from build123d import *

# Parameters (mm, degrees)
SKETCH_1_R      = 3
EXTRUDE_1_DEPTH = 5


with BuildPart() as part:
    # 草图1 → 凸台-拉伸1 (new body)
    with BuildSketch(Plane(origin=(0, 0, 0), x_dir=(1, 0, 0), z_dir=(0, 1, 0))):
        with BuildLine():
            Line((-39.885379482, -89.051728746), (240.960836827, -260.037504895))
            ThreePointArc((240.960836827, -260.037504895), (227.643725358, 34.228528193), (-39.885379482, -89.051728746))
        make_face()
        with Locations(Location((20.435189142, -16.402343887, 0), (0, 0, 270))):
            Circle(SKETCH_1_R, mode=Mode.SUBTRACT)
        with Locations(Location((-9.564810858, -68.363868114, 0), (0, 0, 270))):
            Circle(SKETCH_1_R, mode=Mode.SUBTRACT)
        with Locations(Location((250.242810277, -218.363868114, 0), (0, 0, 270))):
            Circle(SKETCH_1_R, mode=Mode.SUBTRACT)
        with Locations(Location((280.242810277, -166.402343887, 0), (0, 0, 270))):
            Circle(SKETCH_1_R, mode=Mode.SUBTRACT)
    extrude(amount=EXTRUDE_1_DEPTH)


solid = part.part
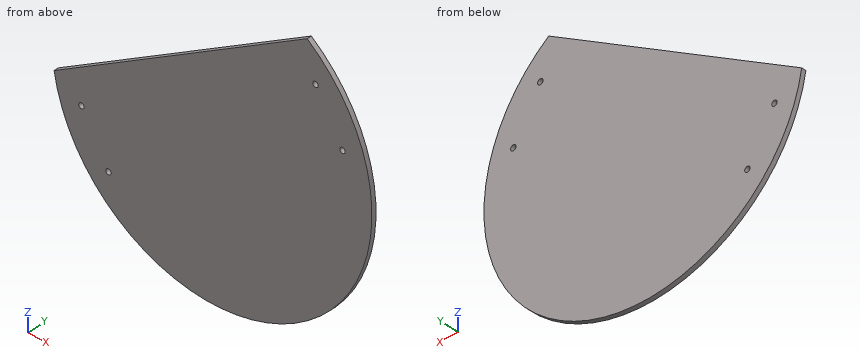
The listing builds one solid part. Answer for the finished solid, in the listing's coordinates (mm). Coordinates: 2 decimals unless noted, no trailing zeros. Loops run counter-clockwise (first coordinate to the right, second up) from the corner with the lowest first, then second, coordinate; pieces in that order, holes last.
1) Flat-ended cylindrical pins translate along their axes: pin 1 Ø2 at (x, y) = (210.5, 4) entering from +Z; pin 2 Ø3 at (x, y) = (146, 2.5) entering from -Z; pin 3 Ø2 at (x, y) = (78.5, 2.5) entering from -Z. Find the tip coordinate at first contact, or state that the pin passes through.
2) Find section A-A on y = 1.75. Write down the section's boundary in (x, z).
3) Find section C-C on z = 104.5. Write down the section's boundary in (x, y), then the cut area to 3 significant figures.
4) Find section B-B on x = 237. Write down the section's boundary in (y, z).
5) Find the intervals of material crossed by L1, parallel to Z at x = 29, y = 1.45; L2, parallel to X at y = 4.3, z = 68.5; L3, parallel to Z at x = 278, y = 1.05, in increasing order.
Values:
1. pin 1: stops at z = 242.1
1. pin 2: stops at z = -59.88
1. pin 3: stops at z = -51.11
2. outline: (-39.89, 89.05) arc R177.5 ccw (long way) to (240.96, 260.04) - close; hole circle Ø6 at (-9.56, 68.36); hole circle Ø6 at (20.44, 16.4); hole circle Ø6 at (250.24, 218.36); hole circle Ø6 at (280.24, 166.4)
3. outline: (-14.51, 0) - (312.37, 0) - (312.37, 5) - (-14.51, 5) - close
3. area: 1,630 mm2
4. outline: (0, -28.12) - (5, -28.12) - (5, 257.63) - (0, 257.63) - close
5. L1: z = -24.74 to 130.99
5. L2: x = -35.3 to -12.56, -6.57 to 305.98
5. L3: z = 11.77 to 164.41, 168.39 to 223
